```python
from build123d import *

# Parameters (mm, degrees)
EXTRUDE_1_DEPTH     = 10
SKETCH_3_W          = 32
SKETCH_3_H          = 2
CUT_EXTRUDE_2_DEPTH = 27.076809621
SKETCH_5_W          = 9
SKETCH_5_H          = 5
EXTRUDE_2_DEPTH     = 10
FILLET_1_R          = 1
SKETCH_6_R          = 1.5
CUT_EXTRUDE_3_DEPTH = 30.086079144
FILLET_2_R          = 4


with BuildPart() as part:
    # 草图1 → 凸台-拉伸1 (new body)
    with BuildSketch(Plane.XY):
        with BuildLine():
            ThreePointArc((-10.75, 0), (0, 10.75), (10.75, 0))
            Line((10.75, 0), (16, 0))
            Line((16, 0), (16, 18))
            Line((16, 18), (-16, 18))
            Line((-16, 18), (-16, 0))
            Line((-16, 0), (-10.75, 0))
        make_face()
    extrude(amount=EXTRUDE_1_DEPTH)

    # 草图3 → 切除-拉伸2 (cut, through all)
    with BuildSketch(Plane.XY.offset(10)):
        with Locations((0, 1)):
            Rectangle(SKETCH_3_W, SKETCH_3_H)
    extrude(amount=-CUT_EXTRUDE_2_DEPTH, mode=Mode.SUBTRACT)

    # 草图5 → 凸台-拉伸2 (add)
    with BuildSketch(Plane.XY.offset(10)):
        with Locations((20.5, 4.5)):
            Rectangle(SKETCH_5_W, SKETCH_5_H)
        with Locations((-20.5, 4.5)):
            Rectangle(SKETCH_5_W, SKETCH_5_H)
    extrude(amount=-EXTRUDE_2_DEPTH)

    # 圆角1
    fillet_1_edges = [part.edges().sort_by_distance(p)[0] for p in [
        (-16, 7, 5),
        (16, 7, 5),
    ]]
    fillet(fillet_1_edges, radius=FILLET_1_R)

    # 草图6 → 切除-拉伸3 (cut, through all)
    with BuildSketch(Plane(origin=(0, 7, 0), x_dir=(1, 0, 0), z_dir=(0, 1, 0))):
        with Locations(Location((21, -5, 0), (0, 0, 180))):
            Circle(SKETCH_6_R)
        with Locations((-21, -5)):
            Circle(SKETCH_6_R)
    extrude(amount=-CUT_EXTRUDE_3_DEPTH, mode=Mode.SUBTRACT)

    # 圆角2
    fillet_2_edges = [part.edges().sort_by_distance(p)[0] for p in [
        (-16, 18, 5),
        (16, 18, 5),
    ]]
    fillet(fillet_2_edges, radius=FILLET_2_R)


solid = part.part
```
The model under review builds one solid part; all positions refer to its coordinate system, in mm. A direction names the side the tool comes from. Give positions to 0.01 mm unless a question says otherwise; leave off trailing zeros. Write each loop counter-clockwise with the first axis right and the second up, starting at its lowest first coordinate (ties: lowest second). Pieces come first, ordered by that corner, then holes.
(1) Consider section A-A, the plane z = 5. Give the boundary of the cut face in (x, y).
(2) Consider section C-C, the plane y = 10.25. Give the boundary of the cut face in (x, z).
(3) For P1, Ø3, axis at y = 13, z = 6, coming from the -X side; P2, Ø4, axis at x = 5, z = 5, coming from the -Y side; P3, Ø4, axis at x = 22.5, z = 5.5, coming from the +Y side, all flat-tipped, find the tip position at first contact; note any pin that passes through.
(4) To check wall thickness, follow L1, parallel to Z at x = 21, y = 3.45; L2, parallel to Y at x = -22, z = 2.25; L3, parallel to X at y = 7.75, z = 8. State the ranges of each line that lie inside material, in increasing order.
(5) Consider section D-D, the plane z = 9.25. Give the boundary of the cut face in (x, y), and give its area (3 significant figures).
(6) Tool access review of faces 4 (the flat face through (16, 11, 5)), 5 (the flat face through (-23, 7, 5)), 6 (the flat face through (18, 2, 5)): name each direction out of +Z, -Z, +X, -X, +Y, -Y from which nothing blocks a thin tool from reaching the whole face with its end or side.
(7) Consider section B-B, the plane x = -21. Give the boundary of the cut face in (y, z), and give its area (3 significant figures).
(8) The part is to be moulded in two halves that separate along X. For faces 1 (the cylindrical face through (22.5, 4.54, 5.07)), 2 (the cylindrical face through (16.285, 7.301, 4.93)), 3 (the flat face through (19, 7, 5)), say which applies: released by +X, released by -X, zero draft, split by the parting line, or undercut.
Returned:
1. outline: (-25, 2) - (-22.5, 2) - (-22.5, 7) - (-25, 7) - close; (-19.5, 2) - (-10.56, 2) arc R10.75 cw to (10.56, 2) - (19.5, 2) - (19.5, 7) - (17, 7) arc R1 cw to (16, 8) - (16, 14) arc R4 ccw to (12, 18) - (-12, 18) arc R4 ccw to (-16, 14) - (-16, 8) arc R1 cw to (-17, 7) - (-19.5, 7) - close; (22.5, 2) - (25, 2) - (25, 7) - (22.5, 7) - close
2. outline: (-16, 0) - (-3.24, 0) - (-3.24, 10) - (-16, 10) - close; (3.24, 0) - (16, 0) - (16, 10) - (3.24, 10) - close
3. P1: stops at x = -16
3. P2: stops at y = 8.16
3. P3: stops at y = 7
4. L1: z = 0 to 3.5, 6.5 to 10
4. L2: y = 2 to 7
4. L3: x = -16.03 to -7.45, 7.45 to 16.03
5. outline: (-25, 2) - (-10.56, 2) arc R10.75 cw to (10.56, 2) - (25, 2) - (25, 7) - (17, 7) arc R1 cw to (16, 8) - (16, 14) arc R4 ccw to (12, 18) - (-12, 18) arc R4 ccw to (-16, 14) - (-16, 8) arc R1 cw to (-17, 7) - (-25, 7) - close
5. area: 457 mm2
6. face 4: +Z, -Z, +X, +Y
6. face 5: +Z, -Z, -X, +Y
6. face 6: +Z, -Z, +X, -X, -Y
7. outline: (2, 0) - (7, 0) - (7, 3.5) - (2, 3.5) - close; (2, 6.5) - (7, 6.5) - (7, 10) - (2, 10) - close
7. area: 35.0 mm2
8. face 1: undercut
8. face 2: released by +X
8. face 3: zero draft
